Autodesk Fusion 360 part; units mm, degrees
sketch "Sketch1" plane through (0, 0, 0) normal (0, 0, 1) x (1, 0, 0)
  line L0 (-84.9, 11.9) -> (84.9, 11.9)
  line L1 (84.9, 11.9) -> (84.9, -11.9)
  line L2 (84.9, -11.9) -> (-84.9, -11.9)
  line L3 (-84.9, -11.9) -> (-84.9, 11.9)
  circle A0 centre (-81.9, 8.9) radius 3
  circle A1 centre (-81.9, -8.9) radius 3
  circle A2 centre (81.9, 8.9) radius 3
  circle A3 centre (81.9, -8.9) radius 3
  line L4 (-107.1873, 0) -> (-105, 0)
  line L5 (-105, 0) -> (105, 0) construction
  circle A4 centre (-81, 0) radius 2.2
  circle A5 centre (81, 0) radius 2.2
  dimension "d21" = 169.8
  dimension "d22" = 84.9
  dimension "d23" = 23.8
  dimension "d24" = 11.9
  dimension "d25" = 6
  dimension "d26" = 6
  dimension "d27" = 6
  dimension "d28" = 6
  dimension "d29" = 210
  dimension "d30" = 4.4
  dimension "d31" = 4.4
  dimension "d32" = 3.9
  dimension "d33" = 3.9
extrude "Extrude1" add sketch "Sketch1" along normal blind 2.8 contours L0 L1 L2 L3 A0 A1 A2 A3 | A0 | A2 | A1 | A3
sketch "Sketch2" plane through (0, 0, 2.8) normal (0, 0, 1) x (-1, 0, 0)
  circle A0 centre (81, 0) radius 2.2
  circle A1 centre (-81, 0) radius 2.2
  arc A2 (81.9, -11.9) -> (84.9, -8.9) centre (81.9, -8.9) ccw
  line L0 (84.9, -8.9) -> (84.9, 8.9)
  arc A3 (84.9, 8.9) -> (81.9, 11.9) centre (81.9, 8.9) ccw
  line L1 (81.9, 11.9) -> (-81.9, 11.9)
  arc A4 (-81.9, 11.9) -> (-84.9, 8.9) centre (-81.9, 8.9) ccw
  line L2 (-84.9, 8.9) -> (-84.9, -8.9)
  arc A5 (-84.9, -8.9) -> (-81.9, -11.9) centre (-81.9, -8.9) ccw
  line L3 (-81.9, -11.9) -> (81.9, -11.9)
  line L4 (-81.9, -13.3) -> (81.9, -13.3)
  arc A6 (81.9, -13.3) -> (86.3, -8.9) centre (81.9, -8.9) ccw
  line L5 (86.3, -8.9) -> (86.3, 8.9)
  arc A7 (86.3, 8.9) -> (81.9, 13.3) centre (81.9, 8.9) ccw
  line L6 (81.9, 13.3) -> (-81.9, 13.3)
  arc A8 (-81.9, 13.3) -> (-86.3, 8.9) centre (-81.9, 8.9) ccw
  line L7 (-86.3, 8.9) -> (-86.3, -8.9)
  arc A9 (-86.3, -8.9) -> (-81.9, -13.3) centre (-81.9, -8.9) ccw
  dimension "d36" = 1.4
extrude "Extrude2" add sketch "Sketch2" along normal blind 1.44 contours A2 L0 A3 L1 A4 L2 A5 L3 | L4 A6 L5 A7 L6 A8 L7 A9
chamfer "Chamfer1" distance 0.6 angle 45 8 edges at (86.3, 0, 4.24) (85.0113, 12.0113, 4.24) (0, 13.3, 4.24) (-85.0113, 12.0113, 4.24) (-86.3, 0, 4.24) (-85.0113, -12.0113, 4.24) (0, -13.3, 4.24) (85.0113, -12.0113, 4.24)
sketch "Sketch4" plane through (-1.7827, -2.3697, 0) normal (0, 0, -1) x (1, 0, 0)
  circle A0 centre (-79.2173, -2.3697) radius 2.2
  circle A1 centre (82.7827, -2.3697) radius 2.2
  arc A2 (-83.1173, -11.2697) -> (-80.1173, -14.2697) centre (-80.1173, -11.2697) ccw
  line L0 (-80.1173, -14.2697) -> (83.6827, -14.2697)
  arc A3 (83.6827, -14.2697) -> (86.6827, -11.2697) centre (83.6827, -11.2697) ccw
  line L1 (86.6827, -11.2697) -> (86.6827, 6.5303)
  arc A4 (86.6827, 6.5303) -> (83.6827, 9.5303) centre (83.6827, 6.5303) ccw
  line L2 (83.6827, 9.5303) -> (-80.1173, 9.5303)
  arc A5 (-80.1173, 9.5303) -> (-83.1173, 6.5303) centre (-80.1173, 6.5303) ccw
  line L3 (-83.1173, 6.5303) -> (-83.1173, -11.2697)
  line L4 (-82.9173, 6.5303) -> (-82.9173, -11.2697)
  arc A6 (-82.9173, -11.2697) -> (-80.1173, -14.0697) centre (-80.1173, -11.2697) ccw
  line L5 (-80.1173, -14.0697) -> (83.6827, -14.0697)
  arc A7 (83.6827, -14.0697) -> (86.4827, -11.2697) centre (83.6827, -11.2697) ccw
  line L6 (86.4827, -11.2697) -> (86.4827, 6.5303)
  arc A8 (86.4827, 6.5303) -> (83.6827, 9.3303) centre (83.6827, 6.5303) ccw
  line L7 (83.6827, 9.3303) -> (-80.1173, 9.3303)
  arc A9 (-80.1173, 9.3303) -> (-82.9173, 6.5303) centre (-80.1173, 6.5303) ccw
  dimension "d44" = -0.2
extrude "Extrude4" cut sketch "Sketch4" against normal up to surface (2.8 mm away) contours A2 L0 A3 L1 A4 L2 A5 L3
equation "d22 = d21 / 2"
equation "d24 = d23 / 2"
equation "d26 = d25"
equation "d27 = d25"
equation "d28 = d25"
equation "d33 = d32"
Read the model definition and answer for the solid it produces. Units are mm, in the model's axes. A direction names the side the tool comes from. Coordinates: 2 decimals unless noted, no trailing zeros. Write each loop counter-clockwise with the first axis right and the second up, starting at its lowest first coordinate (ties: lowest second). Pieces come first, ordered by that corner, then holes. Notation, with made-up numbers: M 37.5,6 L 91.5,6 A16 ccw 91.5,10 Z; hole C 31.25,7.25 d1. An arc over 180 degrees is marked long. Use a Markdown table: item, result.
Q1. Determine the mould class of faces 1 (the face through (1, -11.7, 1)), 2 (the face through (-85.045, 11.977, 3.214)), 3 (the face through (84.977, 12.045, 3.214)) for opening direction X: released by +X, released by -X, zero draft, split by the parting line, or undercut.
Answer block:
| item | result |
|---|---|
| face 1 | zero draft |
| face 2 | released by -X |
| face 3 | released by +X |
Q2. The part is cut by section A-A, the plane x = -17. Write down the section's boundary in (y, z), then the cut area to 3 significant figures.
Answer block:
| item | result |
|---|---|
| outline | M -13.3,2.8 L -11.7,2.8 L -11.7,0 L 11.7,0 L 11.7,2.8 L 13.3,2.8 L 13.3,3.64 L 12.7,4.24 L -12.7,4.24 L -13.3,3.64 Z |
| area | 103 mm2 |
Q3. Straight lines are drawn through the part: L1, parallel to X at y = 0, z = 2.9; L2, parallel to X at y = 0, z = 2.6; L3, parallel to Y at x = -81, z = 2.7. For each, find the intervals that lie inside material, in ascending order. Write a range as [from, to].
Answer block:
| item | result |
|---|---|
| L1 | x = [-86.3, -83.2], [-78.8, 78.8], [83.2, 86.3] |
| L2 | x = [-84.7, -83.2], [-78.8, 78.8], [83.2, 84.7] |
| L3 | y = [-11.7, -2.2], [2.2, 11.7] |
Q4. Which of the six approach directions +Z, -Z, +X, -X, +Y, -Y give full straight-line access (tool end or side, diameter ignored) to faces 4 (the face through (-83.9, 10.86, 1.38)), 5 (the face through (83.86, 10.9, 1.38)), 6 (the face through (-84.7, 0, 1)), 7 (the face through (-83.86, -10.9, 1.38)), 8 (the face through (83.9, -10.86, 1.38))?
Answer block:
| item | result |
|---|---|
| face 4 | -Z, -X, +Y |
| face 5 | -Z, +X, +Y |
| face 6 | -Z, -X, +Y, -Y |
| face 7 | -Z, -X, -Y |
| face 8 | -Z, +X, -Y |
Q5. The part is cut by section B-B, the plane z = 0.95. Write down the section's boundary in (x, y).
Answer block:
| item | result |
|---|---|
| outline | M -84.7,-8.9 A2.8 ccw -81.9,-11.7 L 81.9,-11.7 A2.8 ccw 84.7,-8.9 L 84.7,8.9 A2.8 ccw 81.9,11.7 L -81.9,11.7 A2.8 ccw -84.7,8.9 Z; hole C -81,0 d4.4; hole C 81,0 d4.4 |
Q6. Each of these flat-tipped pins is pushed along its axis until it touches: pin 1 Ø2 at (x, z) = (-28.5, 1.5) entering from -Y; pin 2 Ø0.8 at (x, z) = (35, 2) entering from +Y; pin 3 Ø4 at (x, y) = (81, 0) entering from +Z; pin 4 Ø1.4 at (y, z) = (-2, 1) entering from +X. Where does it stop, or does it pass through?
Answer block:
| item | result |
|---|---|
| pin 1 | stops at y = -11.7 |
| pin 2 | stops at y = 11.7 |
| pin 3 | passes through |
| pin 4 | stops at x = 84.7 |
